Can you work these out from the model? Positions are in its coordinate system, mm. Coordinates: 2 decimals unless noted, no trailing zeros. Write each loop counter-clockwise with the first axis right and the second up, starting at its lowest first coordinate (ties: lowest second). Pieces come first, ordered by that corner, then holes. Notation, with made-up numbers: (68.5, 35) - (77.5, 35) arc R24 cw to (77.5, 63) - close; hole circle Ø9 at (-27, 19.5). An arc over 180 degrees is marked (long way). One line per question, with ' | ' between items. Start each with the question number.
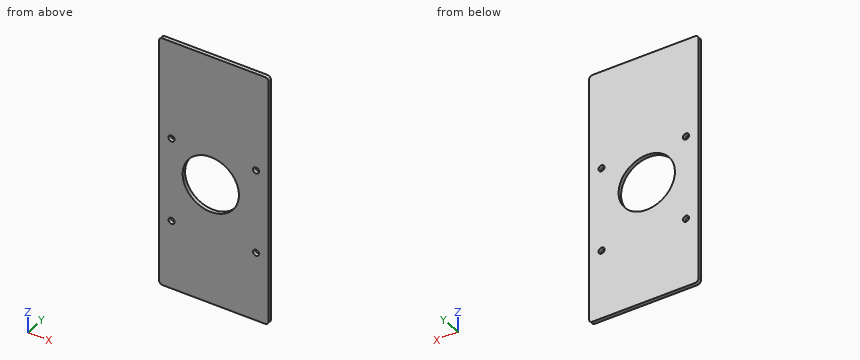
from build123d import *

# Parameters (mm, degrees)
SKETCH1_W           = 58.4
SKETCH1_H           = 134.95
BOSS_EXTRUDE1_DEPTH = 2
FILLET1_R           = 2
SKETCH2_R           = 1.65
CUT_EXTRUDE1_DEPTH  = 101.736235674
SKETCH3_R           = 15
CUT_EXTRUDE2_DEPTH  = 101.736235674


with BuildPart() as part:
    # Sketch1 → Boss-Extrude1 (new body)
    with BuildSketch(Plane(origin=(0, 0, 0), x_dir=(1, 0, 0), z_dir=(0, 1, 0))):
        with Locations((-17.49012047, -21.765247804)):
            Rectangle(SKETCH1_W, SKETCH1_H)
    extrude(amount=BOSS_EXTRUDE1_DEPTH)

    # Fillet1
    fillet1_edges = [part.edges().sort_by_distance(p)[0] for p in [
        (-46.69012047, 1, -45.709752196),
        (11.70987953, 1, -45.709752196),
        (11.70987953, 1, 89.240247804),
        (-46.69012047, 1, 89.240247804),
    ]]
    fillet(fillet1_edges, radius=FILLET1_R)

    # Sketch2 → Cut-Extrude1 (cut, through all)
    with BuildSketch(Plane(origin=(0, 2, 0), x_dir=(1, 0, 0), z_dir=(0, 1, 0))):
        with Locations(Location((-39.99012047, 8.709752196, 0), (0, 0, 270))):
            Circle(SKETCH2_R)
        with Locations(Location((5.00987953, 8.709752196, 0), (0, 0, 270))):
            Circle(SKETCH2_R)
        with Locations(Location((5.00987953, -36.290247804, 0), (0, 0, 270))):
            Circle(SKETCH2_R)
        with Locations(Location((-39.99012047, -36.290247804, 0), (0, 0, 270))):
            Circle(SKETCH2_R)
    extrude(amount=-CUT_EXTRUDE1_DEPTH, mode=Mode.SUBTRACT)

    # Sketch3 → Cut-Extrude2 (cut, through all)
    with BuildSketch(Plane(origin=(0, 2, 0), x_dir=(1, 0, 0), z_dir=(0, 1, 0))):
        with Locations(Location((-19.084532275, -19.290247804, 0), (0, 0, 270))):
            Circle(SKETCH3_R)
    extrude(amount=-CUT_EXTRUDE2_DEPTH, mode=Mode.SUBTRACT)


solid = part.part
(1) If I drill on probe 1 along Z at (x, y) = (-39, 0.65); probe 2 along Z at (x, y) = (-20, 0.9); probe 3 along X at (y, z) = (1.75, 10.5), over which ranges is the centre line in solid material (lowest first)?
(2) If we section it at B-B on z = 18.5: List the corners of the cut face in (x, y) for me, plus the area to 3 significant figures.
(3) If we section it at C-C on y = 1.5: List the corners of the cut face in (x, z) for me.
(4) I'm going to push a flat-ended pin straight in: pin 1 (3 mm diameter, centred on x = -39.99, z = -8.71, fed in from +Y). Where does the tip first touch, or does it pass through?
(5) If we section it at A-A on x = -15.5: List the corners of the cut face in (y, z) for me, plus the area to 3 significant figures.
Values:
1) probe 1: -45.71 to -10.03, -7.39 to 34.97, 37.61 to 89.24 | probe 2: -45.71 to 4.32, 34.26 to 89.24 | probe 3: -46.69 to -31.24, -6.93 to 11.71
2) outline: (-46.69, 0) - (-34.06, 0) - (-34.06, 2) - (-46.69, 2) - close; (-4.11, 0) - (11.71, 0) - (11.71, 2) - (-4.11, 2) - close | area: 56.9 mm2
3) outline: (-46.69, -43.71) arc R2 ccw to (-44.69, -45.71) - (9.71, -45.71) arc R2 ccw to (11.71, -43.71) - (11.71, 87.24) arc R2 ccw to (9.71, 89.24) - (-44.69, 89.24) arc R2 ccw to (-46.69, 87.24) - close; hole circle Ø3.3 at (-39.99, -8.71); hole circle Ø3.3 at (-39.99, 36.29); hole circle Ø30 at (-19.08, 19.29); hole circle Ø3.3 at (5.01, -8.71); hole circle Ø3.3 at (5.01, 36.29)
4) pin 1: through
5) outline: (0, -45.71) - (2, -45.71) - (2, 4.72) - (0, 4.72) - close; (0, 33.86) - (2, 33.86) - (2, 89.24) - (0, 89.24) - close | area: 212 mm2
